Job drawing, mm, ordinate dimensions from the low corner. One solid piece. A direction names the side the tool comes from. Give positions to 0.01 mm unless a question says otherwise; leave off trailing zeros. Write each loop counter-clockwise with the first axis right and the second up, starting at its lowest first coordinate (ties: lowest second). Pieces come first, ordered by that corner, then holes. Notation, with made-up numbers: M -25.75,30.25 L -11.75,30.25 A21 ccw -11.75,54.25 Z; hole C 16,23.5 d10. An arc over 180 degrees is marked long. Answer as CSV lines item,"result". Start each with the question number.
Item 1: Band-saw the part on C-C, the plane z = 11. List the corners of the cut face in (x, y).
Item 2: Wall check: L1, parallel to Y at x = 20.32, z = 19.75; L2, parallel to X at y = 10.16, z = 7; L3, parallel to X at y = 10.16, z = 10.5. Give the ranges that are in metal, low to high. Write a range as from..to.
Item 3: Band-saw the part on B-B, the plane y = 10.75. List the corners of the cut face in (x, z).
Item 4: Two-plate mould, pull along Z, no slides. Class the marked faces 1, 2 and 3: +Z half, -Z half, draft (parallel to the pull), parting line (faces both ways), or undercut.
Item 5: Pin check, flat tips, straight feed: pin 1 (6 mm diameter, centred on x = 20.32, y = 10.16, fed in from -Z); pin 2 (1 mm diameter, centred on y = 0.5, z = 3.5, fed in from +X); pin 3 (12 mm diameter, centred on x = 36.5, z = 19.5, fed in from -Y); pin 4 (0.6 mm diameter, centred on x = 21, y = 0.5, fed in from +Z). Stop position of each tip, or through.
Item 6: Band-saw the part on A-A, the plane x = 18.5. List the corners of the cut face in (y, z), then the cut area to 3 significant figures.
Item 7: 3-axis set-ups, long thin cutter, end or side, ignore diameter. For the marked faces 4 and 5: which of +Z, -Z, +X, -X, +Y, -Y reach the whole face in a straight line?
Item 8: Band-saw the part on D-D, the plane y = 13.25. List the corners of the cut face in (x, z) (1 decimal).
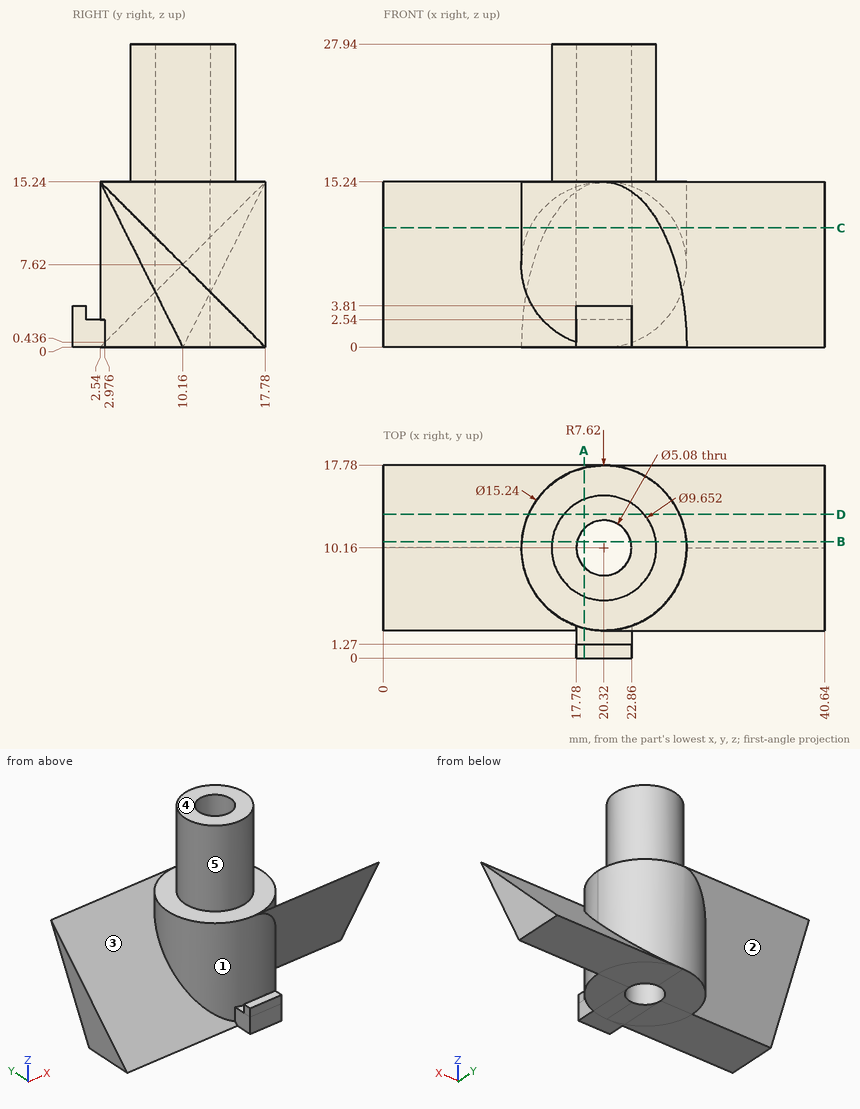
Output:
1,outline,"M 0,13.54 L 13.49,13.54 A7.62 ccw 25.59,4.66 L 40.64,4.66 L 40.64,6.78 L 27.15,6.78 A7.62 ccw 15.05,15.66 L 0,15.66 Z; hole C 20.32,10.16 d5.08"
2,L1,"5.33..7.62, 12.7..14.99"
2,L2,"0..17.78, 22.86..40.64"
2,L3,"12.7..17.78, 22.86..27.94"
3,outline,"M 0,1.18 L 12.72,1.18 L 12.72,0 L 17.85,0 L 17.85,27.94 L 15.53,27.94 L 15.53,15.24 L 12.72,15.24 L 12.72,8.21 L 0,8.21 Z; M 22.79,0 L 40.64,0 L 40.64,7.03 L 27.92,7.03 L 27.92,15.24 L 25.11,15.24 L 25.11,27.94 L 22.79,27.94 Z"
4,face 1,"undercut"
4,face 2,"-Z half"
4,face 3,"+Z half"
5,pin 1,"z = 0"
5,pin 2,"x = 22.86"
5,pin 3,"y = 2.54"
5,pin 4,"z = 3.81"
6,outline,"M 0,0 L 8.39,0 L 8.39,27.94 L 5.69,27.94 L 5.69,15.24 L 2.76,15.24 L 2.76,2.54 L 1.27,2.54 L 1.27,3.81 L 0,3.81 Z; M 11.93,0 L 17.56,0 L 17.56,14.8 L 17.78,15.24 L 17.56,15.02 L 17.56,15.24 L 14.63,15.24 L 14.63,27.94 L 11.93,27.94 Z"
6,area,"249 mm²"
7,face 4,"+Z, +X, -X, +Y, -Y"
7,face 5,"+Z"
8,outline,"M 0,6.2 L 13.4,6.2 L 13.4,0 L 40.6,0 L 40.6,4.5 L 27.3,4.5 L 27.3,15.2 L 24,15.2 L 24,27.9 L 16.6,27.9 L 16.6,15.2 L 13.4,15.2 L 13.4,10.7 L 0,10.7 Z"
